from build123d import *

# Parameters (mm, degrees)
SKETCH4_R           = 2.5
SKETCH4_R_2         = 1.8415
BOSS_EXTRUDE4_DEPTH = 7.5
SKETCH5_W           = 63
SKETCH5_H           = 54
SKETCH5_W_2         = 54.464466094
SKETCH5_H_2         = 45.464466094
BOSS_EXTRUDE5_DEPTH = 2


with BuildPart() as part:
    # Sketch4 → Boss-Extrude4 (new body)
    # profile 1 of 8: a face of its own
    with BuildSketch(Plane(origin=(0, 0, 0), x_dir=(1, 0, 0), z_dir=(0, 1, 0))):
        with Locations(Location((58, 0, 0), (0, 0, 270))):
            Circle(SKETCH4_R)
        with Locations((58, 0)):
            Circle(SKETCH4_R_2, mode=Mode.SUBTRACT)
    # profile 2 of 8: a face of its own
    with BuildSketch(Plane(origin=(0, 0, 0), x_dir=(1, 0, 0), z_dir=(0, 1, 0))):
        with Locations((58, 0)):
            Circle(SKETCH4_R_2)
    # profile 3 of 8: a face of its own
    with BuildSketch(Plane(origin=(0, 0, 0), x_dir=(1, 0, 0), z_dir=(0, 1, 0))):
        with Locations(Location((0, 0, 0), (0, 0, 270))):
            Circle(SKETCH4_R)
        Circle(SKETCH4_R_2, mode=Mode.SUBTRACT)
    # profile 4 of 8: a face of its own
    with BuildSketch(Plane(origin=(0, 0, 0), x_dir=(1, 0, 0), z_dir=(0, 1, 0))):
        Circle(SKETCH4_R_2)
    # profile 5 of 8: a face of its own
    with BuildSketch(Plane(origin=(0, 0, 0), x_dir=(1, 0, 0), z_dir=(0, 1, 0))):
        with Locations(Location((0, 49, 0), (0, 0, 270))):
            Circle(SKETCH4_R)
        with Locations((0, 49)):
            Circle(SKETCH4_R_2, mode=Mode.SUBTRACT)
    # profile 6 of 8: a face of its own
    with BuildSketch(Plane(origin=(0, 0, 0), x_dir=(1, 0, 0), z_dir=(0, 1, 0))):
        with Locations((0, 49)):
            Circle(SKETCH4_R_2)
    # profile 7 of 8: a face of its own
    with BuildSketch(Plane(origin=(0, 0, 0), x_dir=(1, 0, 0), z_dir=(0, 1, 0))):
        with Locations(Location((58, 49, 0), (0, 0, 270))):
            Circle(SKETCH4_R)
        with Locations((58, 49)):
            Circle(SKETCH4_R_2, mode=Mode.SUBTRACT)
    # profile 8 of 8: a face of its own
    with BuildSketch(Plane(origin=(0, 0, 0), x_dir=(1, 0, 0), z_dir=(0, 1, 0))):
        with Locations((58, 49)):
            Circle(SKETCH4_R_2)
    extrude(amount=BOSS_EXTRUDE4_DEPTH)

    # Sketch5 → Boss-Extrude5 (add)
    with BuildSketch(Plane.XZ):
        with Locations((29, -24.5)):
            Rectangle(SKETCH5_W, SKETCH5_H)
        with Locations((29, -24.5)):
            Rectangle(SKETCH5_W_2, SKETCH5_H_2, mode=Mode.SUBTRACT)
    extrude(amount=-BOSS_EXTRUDE5_DEPTH)


solid = part.part
Build history of the part. All positions in model axes, mm. A direction names the side the tool comes from. Coordinates: 2 decimals unless noted, no trailing zeros. Order: outer loops, then holes, each group sorted by start corner. A loop starts at its lowest first (then second) coordinate and runs counter-clockwise, first axis right, second up. Notation, with made-up numbers: (-30, 34.5) - (14, 34.5) arc R14 cw to (14, 47.5) - close; hole circle Ø9 at (72.25, 21.25). An arc over 180 degrees is marked (long way). Write each question's results on one line, items separated by ' | '. Start each with the question number.
Item 1: Mould opens along X. For faces 5 (the face through (57.04, 4.71, -46.69)), 6 (the face through (-2.5, 1, -25)), 7 (the face through (29, 2, 0)), 8 (the face through (29, 0, 0)) say: released by +X, released by -X, zero draft, split by the parting line, or undercut.
Item 2: Wall check: probe 1 along Z at (x, y) = (40, 1.75); probe 2 along X at (y, z) = (0.75, -3); probe 3 along X at (y, z) = (2.25, -49). Give the ranges that are in metal, low to high. Write a range as [from, to].
Item 3: Band-saw the part on C-C on y = 0.75. Write the cut outline in (x, z), and give its area (3 significant figures).
Item 4: Band-saw the part on D-D on y = 5.25. Write the cut outline in (x, z), and give its area (3 significant figures).
Item 5: Flat gauge pins, fed straight in: pin 1 (3.5 mm diameter, centred on x = 58, z = -15.5, fed in from +Y); pin 2 (3 mm diameter, centred on x = 48, z = -44.5, fed in from +Y). Where does each tip first touch, or does it go through?
Item 6: Band-saw the part on A-A on z = -17.5. Write the cut outline in (x, y).
Item 7: Band-saw the part on B-B on x = 39. Write the cut outline in (y, z).
Item 8: Tool access for faces 1 (the face through (56.232, 1, -25)), 2 (the face through (-2, 2, 2)), 3 (the face through (60, 2, 2)), 4 (the face through (-2.44, 4.71, -0.54)): list every direction of +Z, -Z, +X, -X, +Y, -Y with a clear straight run to the whole face (end or side of a thin tool).
Numbers:
1) face 5: undercut | face 6: released by -X | face 7: undercut | face 8: zero draft
2) probe 1: [-51.5, -47.23], [-1.77, 2.5] | probe 2: [-2.5, 1.77], [56.23, 60.5] | probe 3: [-2.5, 2.5], [55.5, 60.5]
3) outline: (-2.5, -51.5) - (60.5, -51.5) - (60.5, 2.5) - (-2.5, 2.5) - close; hole (1.77, -47.23) - (56.23, -47.23) - (56.23, -1.77) - (1.77, -1.77) - close | area: 926 mm^2
4) outline: circle Ø5 at (0, -49); circle Ø5 at (0, 0); circle Ø5 at (58, -49); circle Ø5 at (58, 0) | area: 78.5 mm^2
5) pin 1: y = 2 | pin 2: through
6) outline: (-2.5, 0) - (1.77, 0) - (1.77, 2) - (-2.5, 2) - close; (56.23, 0) - (60.5, 0) - (60.5, 2) - (56.23, 2) - close
7) outline: (0, -51.5) - (2, -51.5) - (2, -47.23) - (0, -47.23) - close; (0, -1.77) - (2, -1.77) - (2, 2.5) - (0, 2.5) - close
8) face 1: +Y, -Y | face 2: +Z, -X, +Y | face 3: +Z, +X, +Y | face 4: +Y
